from build123d import *

# Parameters (mm, degrees)
SKETCH_2_R          = 5
EXTRUDE_2_DEPTH     = 30
CUT_EXTRUDE_1_DEPTH = 31.822070015
CUT_EXTRUDE_START   = -3.6000001
CUT_EXTRUDE_2_DEPTH = 3.6000001


# Read off the part's stored shape, not the designer's step: the extrude step
with BuildPart() as part:
    # Sketch 2 → Extrude 2 (new body)
    with BuildSketch(Plane(origin=(0, 0, 0), x_dir=(1, 0, 0), z_dir=(0, 1, 0))):
        with Locations(Location((0, 0, 0), (0, 0, 270))):
            Circle(SKETCH_2_R)
    extrude(amount=EXTRUDE_2_DEPTH)

    # Sketch 4 → Cut-Extrude 1 (cut, through all)
    with BuildSketch(Plane(origin=(0, 30, 0), x_dir=(1, 0, 0), z_dir=(0, 1, 0))):
        with BuildLine():
            Line((0, 1.4), (-1.428285686, 1.4))
            ThreePointArc((-1.428285686, 1.4), (-0.756117924, -1.851563039), (2, 0))
            ThreePointArc((2, 0), (1.851563039, 0.756117924), (1.428285686, 1.4))
            Line((1.428285686, 1.4), (0, 1.4))
        make_face()
    extrude(amount=-CUT_EXTRUDE_1_DEPTH, mode=Mode.SUBTRACT)

    # Cut-Extrude 2 outline → Cut-Extrude 2 (cut)
    with BuildSketch(Plane.XY.offset(-1.4).offset(CUT_EXTRUDE_START)):
        with BuildLine():
            ThreePointArc((-1.428285686, 26.210947143), (0, 25.169204712), (1.428285686, 26.210947143))
            Line((1.428285686, 26.210947143), (1.428285686, 27.127462282))
            ThreePointArc((1.428285686, 27.127462282), (0, 28.169204712), (-1.428285686, 27.127462282))
            Line((-1.428285686, 27.127462282), (-1.428285686, 26.210947143))
        make_face()
    extrude(amount=CUT_EXTRUDE_2_DEPTH, mode=Mode.SUBTRACT)


solid = part.part
Check sheet for the modelled part. Datum: model origin and axes. Units: mm. A direction names the side the tool comes from. Round coordinates to 2 decimals unless told otherwise and drop trailing zeros. Loops run counter-clockwise (first coordinate to the right, second up) from the corner with the lowest first, then second, coordinate; pieces in that order, holes last. Notation, with made-up numbers: M -14.5,45 L 27.5,45 A23 ccw 27.5,78 Z; hole C 0.5,29 d10. An arc over 180 degrees is marked long. One line per question, with ' | ' between items. Start each with the question number.
Item 1: Set-up check for faces 5 (the face through (0.03, 28.17, -3.23)), 6 (the face through (0, 29, -1.4)), 7 (the face through (0.1, 0, 2.2)): record each of +Z, -Z, +X, -X, +Y, -Y from which the full face is reachable in a straight line by a thin tool's end or side.
Item 2: Section check B-B (z = -3.5). Record the boundary of the cut face in (x, y).
Item 3: Release check for a two-part mould opening along Y. For faces 1 (the face through (0, 13, -1.4)), 2 (the face through (-1.428, 26.7, -3.1)), 3 (the face through (0.1, 30, 2.2)), 4 (the face through (1.428, 26.7, -3.1)) record: released by +Y, released by -Y, zero draft, split by the parting line, or undercut.
Item 4: Gauge pin test, flat ends, axial feed: pin 1 Ø0.7 at (y, z) = (26.5, -2.5) entering from +X; pin 2 Ø4 at (y, z) = (7, 3.5) entering from +X; pin 3 Ø1 at (y, z) = (27, -3) entering from +X. Record the tip position at first contact, or that the pin passes through.
Item 5: Section check D-D (x = 3). Record the boundary of the cut face in (y, z), and give its area (3 significant figures).
Item 6: Scan lines: probe 1 along Z at (x, y) = (0, 9); probe 2 along X at (y, z) = (4.5, 0); probe 3 along X at (y, z) = (28, 0.75). Record each from-to range of solid material in increasing order.
Item 7: Section check A-A (x = 0). Record the boundary of the cut face in (y, z).
Item 8: Section check C-C (y = 9). Record the boundary of the cut face in (x, z).
Worked out:
1) face 5: -Z | face 6: +Y, -Y | face 7: +Z, -Z, +X, -X, -Y
2) outline: M -3.57,0 L 3.57,0 L 3.57,30 L -3.57,30 Z; hole M -1.43,26.21 A1.5 ccw 1.43,26.21 L 1.43,27.13 A1.5 ccw -1.43,27.13 Z
3) face 1: zero draft | face 2: undercut | face 3: released by +Y | face 4: undercut
4) pin 1: x = 4.51 | pin 2: x = 4.77 | pin 3: x = 4.33
5) outline: M 0,-4 L 30,-4 L 30,4 L 0,4 Z | area: 240 mm^2
6) probe 1: -5 to -1.4, 2 to 5 | probe 2: -5 to -2, 2 to 5 | probe 3: -4.94 to -1.85, 1.85 to 4.94
7) outline: M 0,-5 L 25.17,-5 L 25.17,-1.4 L 0,-1.4 Z; M 0,2 L 30,2 L 30,5 L 0,5 Z; M 28.17,-5 L 30,-5 L 30,-1.4 L 28.17,-1.4 Z
8) outline: C 0,0 d10; hole M -1.43,-1.4 L 1.43,-1.4 A2 ccw long Z
